from build123d import *

# Parameters (mm, degrees)
SKETCH1_W           = 100
SKETCH1_H           = 100
SKETCH1_R           = 4
BOSS_EXTRUDE1_DEPTH = 25
SKETCH2_R           = 3.6
CUT_EXTRUDE1_DEPTH  = 20
FILLET1_R           = 5
CUT_EXTRUDE3_START  = 17
SKETCH1_3_R         = 7
CUT_EXTRUDE3_DEPTH  = 8


with BuildPart() as part:
    # Sketch1 → Boss-Extrude1 (new body)
    with BuildSketch(Plane(origin=(0, 0, 0), x_dir=(1, 0, 0), z_dir=(0, 1, 0))):
        with Locations((50, 50)):
            Rectangle(SKETCH1_W, SKETCH1_H)
        with Locations(Location((10.606601718, 89.393398282, 0), (0, 0, 270))):
            Circle(SKETCH1_R, mode=Mode.SUBTRACT)
        with Locations(Location((89.393398282, 89.393398282, 0), (0, 0, 270))):
            Circle(SKETCH1_R, mode=Mode.SUBTRACT)
        with Locations(Location((89.393398282, 10.606601718, 0), (0, 0, 270))):
            Circle(SKETCH1_R, mode=Mode.SUBTRACT)
        with Locations(Location((10.606601718, 10.606601718, 0), (0, 0, 270))):
            Circle(SKETCH1_R, mode=Mode.SUBTRACT)
    extrude(amount=BOSS_EXTRUDE1_DEPTH)

    # Sketch2 → Cut-Extrude1 (cut)
    with BuildSketch(Plane.XY):
        with Locations((20, 12.5)):
            Circle(SKETCH2_R)
        with Locations((80, 12.5)):
            Circle(SKETCH2_R)
    extrude(amount=-CUT_EXTRUDE1_DEPTH, mode=Mode.SUBTRACT)

    # Fillet1
    fillet1_edges = [part.edges().sort_by_distance(p)[0] for p in [
        (100, 12.5, -100),
        (0, 12.5, -100),
    ]]
    fillet(fillet1_edges, radius=FILLET1_R)

    # Sketch1<3> → Cut-Extrude3 (cut)
    with BuildSketch(Plane(origin=(0, 0, 0), x_dir=(1, 0, 0), z_dir=(0, 1, 0)).offset(CUT_EXTRUDE3_START)):
        with Locations(Location((10.606601718, 89.393398282, 0), (0, 0, 90))):
            Circle(SKETCH1_3_R)
        with Locations(Location((89.393398282, 89.393398282, 0), (0, 0, 90))):
            Circle(SKETCH1_3_R)
        with Locations(Location((10.606601718, 10.606601718, 0), (0, 0, 90))):
            Circle(SKETCH1_3_R)
        with Locations(Location((89.393398282, 10.606601718, 0), (0, 0, 90))):
            Circle(SKETCH1_3_R)
    extrude(amount=CUT_EXTRUDE3_DEPTH, mode=Mode.SUBTRACT)


solid = part.part
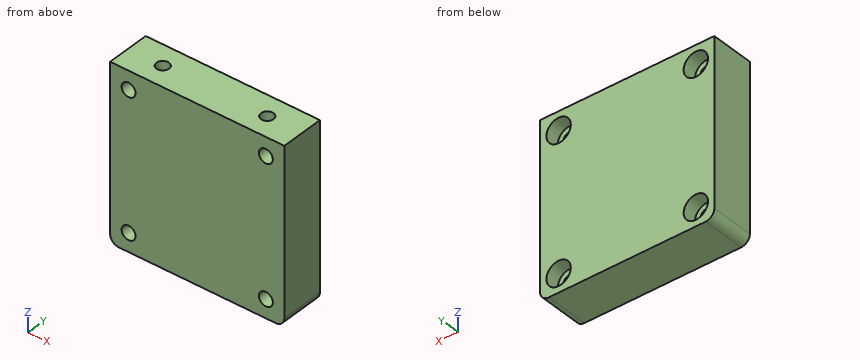
Source: CAD feature listing. Evaluate the final solid. Frame: model axes, mm. Give positions to 0.01 mm unless a question says otherwise; leave off trailing zeros. Loops run counter-clockwise (first coordinate to the right, second up) from the corner with the lowest first, then second, coordinate; pieces in that order, holes last. Notation, with made-up numbers: (54, -22) -> (84, -22) arc R20 cw to (84, 5) -> close; hole circle Ø5 at (74.25, 69.5). An arc over 180 degrees is marked (long way). Use a Markdown table: item, result. Add a question column.
1) First-contact query: pin 1 (5 mm diameter, centred on x = 89.39, z = -10.61, fed in from -Y); pin 2 (7 mm diameter, centred on x = 89, z = -92.5, fed in from +Y); pin 3 (16 mm diameter, centred on x = 89.39, z = -10.61, fed in from -Y). Flat tips, straight axial feed; report the tip coordinate or a pass-through.
2) Line query: line 1 along Z through (x, y) = (89, 4.5); line 2 along X through (y, z) = (17.25, -89.5); line 3 along Z through (x, y) = (88, 6). Output: solid intervals per line, ascending. Write a range as [from, to].
3) Section query C-C, the plane y = 4.25. Return the cut outline in (x, z).
4) Section query D-D, the plane y = 12.5. Return the cut outline in (x, z), then the cut area to 3 significant figures.
5) Section query B-B, the plane x = 80. Return the cut outline in (y, z).
6) Section query A-A, the plane z = -13. Return the cut outline in (x, y), then the cut area to 3 significant figures.
Numbers:
| question | item | result |
|---|---|---|
| 1 | pin 1 | passes through |
| 1 | pin 2 | stops at y = 17 |
| 1 | pin 3 | stops at y = 0 |
| 2 | line 1 | z = [-100, -93.37], [-85.41, -14.59], [-6.63, 0] |
| 2 | line 2 | x = [0, 3.61], [17.61, 82.39], [96.39, 100] |
| 2 | line 3 | z = [-100, -93.14], [-85.64, -14.36], [-6.86, 0] |
| 3 | outline | (0, -95) arc R5 ccw to (5, -100) -> (95, -100) arc R5 ccw to (100, -95) -> (100, 0) -> (0, 0) -> close; hole circle Ø8 at (10.61, -89.39); hole circle Ø8 at (10.61, -10.61); hole circle Ø8 at (89.39, -89.39); hole circle Ø8 at (89.39, -10.61) |
| 4 | outline | (0, -95) arc R5 ccw to (5, -100) -> (95, -100) arc R5 ccw to (100, -95) -> (100, 0) -> (83.6, 0) -> (83.6, -20) -> (76.4, -20) -> (76.4, 0) -> (23.6, 0) -> (23.6, -20) -> (16.4, -20) -> (16.4, 0) -> (0, 0) -> close; hole circle Ø8 at (10.61, -89.39); hole circle Ø8 at (10.61, -10.61); hole circle Ø8 at (89.39, -89.39); hole circle Ø8 at (89.39, -10.61) |
| 4 | area | 9,500 mm2 |
| 5 | outline | (0, -100) -> (25, -100) -> (25, 0) -> (16.1, 0) -> (16.1, -20) -> (8.9, -20) -> (8.9, 0) -> (0, 0) -> close |
| 6 | outline | (0, 0) -> (7.4, 0) -> (7.4, 17) -> (4.03, 17) -> (4.03, 25) -> (0, 25) -> close; (13.81, 0) -> (86.19, 0) -> (86.19, 17) -> (82.82, 17) -> (82.82, 25) -> (17.18, 25) -> (17.18, 17) -> (13.81, 17) -> close; (92.6, 0) -> (100, 0) -> (100, 25) -> (95.97, 25) -> (95.97, 17) -> (92.6, 17) -> close; hole circle Ø7.2 at (20, 12.5); hole circle Ø7.2 at (80, 12.5) |
| 6 | area | 1,990 mm2 |
